Input: part model. Units: mm. Frame: model coordinates. A direction names the side the tool comes from. Give positions to 0.01 mm unless a question says otherwise; leave off trailing zeros. Loops run counter-clockwise (first coordinate to the right, second up) from the corner with the lowest first, then second, coordinate; pieces in that order, holes last. Notation, with made-up numbers: (-15.5, 56) - (15.5, 56) arc R9 ccw to (15.5, 62) - close; hole circle Ø5 at (35, 32.5). An arc over 180 degrees is marked (long way). Answer as a JSON object with one key per item and string values. Group by question number.
(1) Material intervals for L1, parallel to X at y = -7, z = 13.5; L2, parallel to X at y = -2, z = 15.5; L3, parallel to Z at x = -2, y = -1.25, sorted ascending.
(2) Section query A-A (x = -2.5). Return loops of the section in (y, z).
(3) Pin query (flat end, axial travel): P1, Ø1, axis at x = -12, y = -2, coming from the +Z side; P2, Ø4, axis at y = -3, z = -15.5, coming from the +X side; P3, Ø3, axis at y = -5.5, z = 2.5, coming from the +X side. Return the tip coordinate at first contact, or that it passes through.
(4) Section query C-C (x = 17). Return loops of the section in (y, z).
(5) Section query B-B (y = -6). Return loops of the section in (x, z) (3 decimals), plus the area to 3 significant figures.
(6) Access query for faces 4 (the flat face through (-16.74, -3.76, -7.55)), 5 (the flat face through (-2.03, -3.76, 18.2)), 6 (the flat face through (-2.33, -3.757, -18.036)), 7 (the flat face through (16.74, -3.76, 7.55)), 8 (the flat face through (9.11, -3.76, 15.95)). Directions: +Z, -Z, +X, -X, +Y, -Y. A direction counts if a zero-diameter tool reaches every point of the face in a straight line with its end or side. Return the directions, or none.
(7) Mould query, pull axis X, two halves, no side actions, for faces 1 (the flat face through (-8.72, -3.76, 15.96)), 2 (the flat face through (16.43, -3.76, -7.79)), 3 (the flat face through (-12.486, -3.757, -13.222)). Classes: +X half, -X half, draft (parallel to the pull), parting line (faces both ways), or undercut.
(8) Section query D-D (z = 21). Return loops of the section in (x, y).
```python
from build123d import *

# Parameters (mm, degrees)
F0_R     = 1.905
F1_DEPTH = 7.62


with BuildPart() as f1:
    # F0 (on Front) → F1 (new body)
    with BuildSketch(Plane.XZ):
        with BuildLine():
            ThreePointArc((12.6683750064, 0.8956978825), (12.6920912891, 0.4481280054), (12.7, 0))
            ThreePointArc((12.7, 0), (12.6742535258, -0.8082682494), (12.597118494, -1.6132593244))
            Line((12.597118494, -1.6132593244), (14.0147271976, -0.2774704496))
            Line((14.0147271976, -0.2774704496), (12.6683750064, 0.8956978825))
        make_face()
        with BuildLine():
            ThreePointArc((11.1395329808, 6.0992462624), (12.1849640795, 3.5800349694), (12.6683750064, 0.8956978825))
            Line((12.6683750064, 0.8956978825), (14.0147271976, -0.2774704496))
            Line((14.0147271976, -0.2774704496), (21.8401513968, 7.0962953575))
            Line((21.8401513968, 7.0962953575), (11.5012455126, 8.0131716525))
            Line((11.5012455126, 8.0131716525), (11.1395329808, 6.0992462624))
        make_face()
        with BuildLine():
            Line((14.0147271976, -0.2774704496), (12.597118494, -1.6132593244))
            ThreePointArc((12.597118494, -1.6132593244), (11.9621347738, -4.2658330549), (10.7754086772, -6.7216491905))
            Line((10.7754086772, -6.7216491905), (11.1750594361, -8.4621282708))
            Line((11.1750594361, -8.4621282708), (21.8401513968, -7.0962953575))
            Line((21.8401513968, -7.0962953575), (14.0147271976, -0.2774704496))
        make_face()
        with BuildLine():
            ThreePointArc((9.7224526655, 8.1709188081), (10.4822978426, 7.1701765626), (11.1395329808, 6.0992462624))
            Line((11.1395329808, 6.0992462624), (11.5012455126, 8.0131716525))
            Line((11.5012455126, 8.0131716525), (9.7224526655, 8.1709188081))
        make_face()
        with BuildLine():
            Line((11.1750594361, -8.4621282708), (10.7754086772, -6.7216491905))
            ThreePointArc((10.7754086772, -6.7216491905), (10.0584513163, -7.7535512584), (9.2430329028, -8.709554682))
            Line((9.2430329028, -8.709554682), (11.1750594361, -8.4621282708))
        make_face()
        with BuildLine():
            ThreePointArc((5.4270244878, 11.4820470827), (7.7535512584, 10.0584513163), (9.7224526655, 8.1709188081))
            Line((9.7224526655, 8.1709188081), (11.5012455126, 8.0131716525))
            Line((11.5012455126, 8.0131716525), (13.4979558827, 18.5783424402))
            Line((13.4979558827, 18.5783424402), (4.5946789547, 13.243054541))
            Line((4.5946789547, 13.243054541), (5.4270244878, 11.4820470827))
        make_face()
        with BuildLine():
            Line((11.1750594361, -8.4621282708), (9.2430329028, -8.709554682))
            ThreePointArc((9.2430329028, -8.709554682), (7.1701765626, -10.4822978426), (4.7666024759, -11.7715547332))
            Line((4.7666024759, -11.7715547332), (4.0668987964, -13.4145407097))
            Line((4.0668987964, -13.4145407097), (13.4979558827, -18.5783424402))
            Line((13.4979558827, -18.5783424402), (11.1750594361, -8.4621282708))
        make_face()
        with BuildLine():
            ThreePointArc((3.0628838603, 12.3251264683), (4.2658330549, 11.9621347738), (5.4270244878, 11.4820470827))
            Line((5.4270244878, 11.4820470827), (4.5946789547, 13.243054541))
            Line((4.5946789547, 13.243054541), (3.0628838603, 12.3251264683))
        make_face()
        with BuildLine():
            Line((4.0668987964, -13.4145407097), (4.7666024759, -11.7715547332))
            ThreePointArc((4.7666024759, -11.7715547332), (3.5800349694, -12.1849640795), (2.3584229018, -12.4790961779))
            Line((2.3584229018, -12.4790961779), (4.0668987964, -13.4145407097))
        make_face()
        with BuildLine():
            ThreePointArc((-2.3584229018, 12.4790961779), (0.3605453902, 12.6948811346), (3.0628838603, 12.3251264683))
            Line((3.0628838603, 12.3251264683), (4.5946789547, 13.243054541))
            Line((4.5946789547, 13.243054541), (0.0568578782, 22.8437989952))
            ThreePointArc((0.0568578782, 22.8437989952), (0.0027938397, 22.8432910784), (-0.0512710089, 22.8437038472))
            Line((-0.0512710089, 22.8437038472), (-4.0668987964, 13.4145407097))
            Line((-4.0668987964, 13.4145407097), (-2.3584229018, 12.4790961779))
        make_face()
        with BuildLine():
            Line((4.0668987964, -13.4145407097), (2.3584229018, -12.4790961779))
            ThreePointArc((2.3584229018, -12.4790961779), (-0.3605453902, -12.6948811346), (-3.0628838603, -12.3251264683))
            Line((-3.0628838603, -12.3251264683), (-4.5946789547, -13.243054541))
            Line((-4.5946789547, -13.243054541), (0, -22.9640941654))
            Line((0, -22.9640941654), (4.0668987964, -13.4145407097))
        make_face()
        with BuildLine():
            ThreePointArc((-4.7666024759, 11.7715547332), (-3.5800349694, 12.1849640795), (-2.3584229018, 12.4790961779))
            Line((-2.3584229018, 12.4790961779), (-4.0668987964, 13.4145407097))
            Line((-4.0668987964, 13.4145407097), (-4.7666024759, 11.7715547332))
        make_face()
        with BuildLine():
            ThreePointArc((-0.0512710089, 22.8437038472), (0.0027938397, 22.8432910784), (0.0568578782, 22.8437989952))
            Line((0.0568578782, 22.8437989952), (0, 22.9640941654))
            Line((0, 22.9640941654), (-0.0512710089, 22.8437038472))
        make_face()
        with BuildLine():
            Line((0, 22.9640941654), (0.0568578782, 22.8437989952))
            ThreePointArc((0.0568578782, 22.8437989952), (2.2650771249, 23.7934189274), (3.175, 26.0182898492))
            ThreePointArc((3.175, 26.0182898492), (-2.2268632139, 28.281408323), (-0.0512710089, 22.8437038472))
            Line((-0.0512710089, 22.8437038472), (0, 22.9640941654))
        make_face()
        with Locations((0, 26.0182898492)):
            Circle(F0_R, mode=Mode.SUBTRACT)
        with BuildLine():
            Line((-4.5946789547, -13.243054541), (-3.0628838603, -12.3251264683))
            ThreePointArc((-3.0628838603, -12.3251264683), (-4.2658330549, -11.9621347738), (-5.4270244878, -11.4820470827))
            Line((-5.4270244878, -11.4820470827), (-4.5946789547, -13.243054541))
        make_face()
        with BuildLine():
            ThreePointArc((-9.2430329028, 8.709554682), (-7.1701765626, 10.4822978426), (-4.7666024759, 11.7715547332))
            Line((-4.7666024759, 11.7715547332), (-4.0668987964, 13.4145407097))
            Line((-4.0668987964, 13.4145407097), (-13.4979558827, 18.5783424402))
            Line((-13.4979558827, 18.5783424402), (-11.1750594361, 8.4621282708))
            Line((-11.1750594361, 8.4621282708), (-9.2430329028, 8.709554682))
        make_face()
        with BuildLine():
            Line((-4.5946789547, -13.243054541), (-5.4270244878, -11.4820470827))
            ThreePointArc((-5.4270244878, -11.4820470827), (-7.7535512584, -10.0584513163), (-9.7224526655, -8.1709188081))
            Line((-9.7224526655, -8.1709188081), (-11.5012455126, -8.0131716525))
            Line((-11.5012455126, -8.0131716525), (-13.4979558827, -18.5783424402))
            Line((-13.4979558827, -18.5783424402), (-4.5946789547, -13.243054541))
        make_face()
        with BuildLine():
            ThreePointArc((-10.7754086772, 6.7216491905), (-10.0584513163, 7.7535512584), (-9.2430329028, 8.709554682))
            Line((-9.2430329028, 8.709554682), (-11.1750594361, 8.4621282708))
            Line((-11.1750594361, 8.4621282708), (-10.7754086772, 6.7216491905))
        make_face()
        with BuildLine():
            Line((-11.5012455126, -8.0131716525), (-9.7224526655, -8.1709188081))
            ThreePointArc((-9.7224526655, -8.1709188081), (-10.4822978426, -7.1701765626), (-11.1395329808, -6.0992462624))
            Line((-11.1395329808, -6.0992462624), (-11.5012455126, -8.0131716525))
        make_face()
        with BuildLine():
            ThreePointArc((-12.597118494, 1.6132593244), (-11.9621347738, 4.2658330549), (-10.7754086772, 6.7216491905))
            Line((-10.7754086772, 6.7216491905), (-11.1750594361, 8.4621282708))
            Line((-11.1750594361, 8.4621282708), (-21.8401513968, 7.0962953575))
            Line((-21.8401513968, 7.0962953575), (-14.0147271976, 0.2774704496))
            Line((-14.0147271976, 0.2774704496), (-12.597118494, 1.6132593244))
        make_face()
        with BuildLine():
            Line((-11.5012455126, -8.0131716525), (-11.1395329808, -6.0992462624))
            ThreePointArc((-11.1395329808, -6.0992462624), (-12.1849640795, -3.5800349694), (-12.6683750064, -0.8956978825))
            Line((-12.6683750064, -0.8956978825), (-14.0147271976, 0.2774704496))
            Line((-14.0147271976, 0.2774704496), (-21.8401513968, -7.0962953575))
            Line((-21.8401513968, -7.0962953575), (-11.5012455126, -8.0131716525))
        make_face()
        with BuildLine():
            ThreePointArc((-12.6683750064, -0.8956978825), (-12.6948811346, 0.3605453902), (-12.597118494, 1.6132593244))
            Line((-12.597118494, 1.6132593244), (-14.0147271976, 0.2774704496))
            Line((-14.0147271976, 0.2774704496), (-12.6683750064, -0.8956978825))
        make_face()
        with BuildLine():
            ThreePointArc((12.597118494, -1.6132593244), (12.6742535258, -0.8082682494), (12.7, 0))
            ThreePointArc((12.7, 0), (12.6920912891, 0.4481280054), (12.6683750064, 0.8956978825))
            ThreePointArc((12.6683750064, 0.8956978825), (12.1849640795, 3.5800349694), (11.1395329808, 6.0992462624))
            ThreePointArc((11.1395329808, 6.0992462624), (10.4822978426, 7.1701765626), (9.7224526655, 8.1709188081))
            ThreePointArc((9.7224526655, 8.1709188081), (7.7535512584, 10.0584513163), (5.4270244878, 11.4820470827))
            ThreePointArc((5.4270244878, 11.4820470827), (4.2658330549, 11.9621347738), (3.0628838603, 12.3251264683))
            ThreePointArc((3.0628838603, 12.3251264683), (0.3605453902, 12.6948811346), (-2.3584229018, 12.4790961779))
            ThreePointArc((-2.3584229018, 12.4790961779), (-3.5800349694, 12.1849640795), (-4.7666024759, 11.7715547332))
            ThreePointArc((-4.7666024759, 11.7715547332), (-7.1701765626, 10.4822978426), (-9.2430329028, 8.709554682))
            ThreePointArc((-9.2430329028, 8.709554682), (-10.0584513163, 7.7535512584), (-10.7754086772, 6.7216491905))
            ThreePointArc((-10.7754086772, 6.7216491905), (-11.9621347738, 4.2658330549), (-12.597118494, 1.6132593244))
            ThreePointArc((-12.597118494, 1.6132593244), (-12.6948811346, 0.3605453902), (-12.6683750064, -0.8956978825))
            ThreePointArc((-12.6683750064, -0.8956978825), (-12.1849640795, -3.5800349694), (-11.1395329808, -6.0992462624))
            ThreePointArc((-11.1395329808, -6.0992462624), (-10.4822978426, -7.1701765626), (-9.7224526655, -8.1709188081))
            ThreePointArc((-9.7224526655, -8.1709188081), (-7.7535512584, -10.0584513163), (-5.4270244878, -11.4820470827))
            ThreePointArc((-5.4270244878, -11.4820470827), (-4.2658330549, -11.9621347738), (-3.0628838603, -12.3251264683))
            ThreePointArc((-3.0628838603, -12.3251264683), (-0.3605453902, -12.6948811346), (2.3584229018, -12.4790961779))
            ThreePointArc((2.3584229018, -12.4790961779), (3.5800349694, -12.1849640795), (4.7666024759, -11.7715547332))
            ThreePointArc((4.7666024759, -11.7715547332), (7.1701765626, -10.4822978426), (9.2430329028, -8.709554682))
            ThreePointArc((9.2430329028, -8.709554682), (10.0584513163, -7.7535512584), (10.7754086772, -6.7216491905))
            ThreePointArc((10.7754086772, -6.7216491905), (11.9621347738, -4.2658330549), (12.597118494, -1.6132593244))
        make_face()
    extrude(amount=F1_DEPTH)


solid = f1.part
```
Recorded:
{
 "1": {"L1": "x = -12.33 to -4.22, -4.03 to 4.47, 5.02 to 12.54", "L2": "x = -12.79 to -7.88, -3.18 to 3.53, 8.36 to 12.92", "L3": "z = -18.73 to 18.27, 23.55 to 28.48"},
 "2": {"outline": "(-7.62, -17.67) - (0, -17.67) - (0, 17.09) - (-7.62, 17.09) - close; (-7.62, 24.06) - (0, 24.06) - (0, 27.98) - (-7.62, 27.98) - close"},
 "3": {"P1": "stops at z = 18.03", "P2": "stops at x = 13.25", "P3": "stops at x = 18.55"},
 "4": {"outline": "(-7.62, -7.72) - (0, -7.72) - (0, -2.88) - (-7.62, -2.88) - close; (-7.62, 2.54) - (0, 2.54) - (0, 7.53) - (-7.62, 7.53) - close"},
 "5": {"outline": "(-21.84, -7.096) - (-11.501, -8.013) - (-13.498, -18.578) - (-4.595, -13.243) - (0, -22.964) - (4.067, -13.415) - (13.498, -18.578) - (11.175, -8.462) - (21.84, -7.096) - (14.015, -0.277) - (21.84, 7.096) - (11.501, 8.013) - (13.498, 18.578) - (4.595, 13.243) - (0.057, 22.844) arc R3.175 ccw (long way) to (-0.051, 22.844) - (-4.067, 13.415) - (-13.498, 18.578) - (-11.175, 8.462) - (-21.84, 7.096) - (-14.015, 0.277) - close; hole circle Ø3.81 at (0, 26.018)", "area": "1,010 mm^2"},
 "6": {"face 4": "-X, +Y, -Y", "face 5": "+Y, -Y", "face 6": "-Z, +Y, -Y", "face 7": "+X, +Y, -Y", "face 8": "+Z, +Y, -Y"},
 "7": {"face 1": "undercut", "face 2": "+X half", "face 3": "-X half"},
 "8": {"outline": "(-0.84, -7.62) - (0.93, -7.62) - (0.93, 0) - (-0.84, 0) - close"}
}
